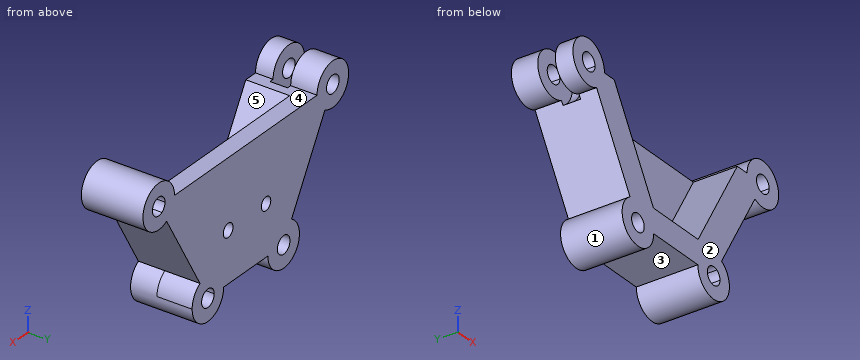
from build123d import *

# Parameters (mm, degrees)
F1_DEPTH  = 50.8
F3_DEPTH  = 76.2
F4_R      = 38.1
F1_FACE_R = 12.7
F5_DEPTH  = 12.7
F6_R      = 9.525
F6_R_2    = 9.7843029872
F7_DEPTH  = 25.401


with BuildPart() as f1:
    # F0 (on Front) → F1 (new body, symmetric)
    with BuildSketch(Plane.XZ):
        with BuildLine():
            ThreePointArc((-130.8751894546, 96.1189323328), (-190.1214960247, 111.9939323328), (-146.7501894546, 68.6226257627))
            Line((-146.7501894546, 68.6226257627), (-156.2751894546, 85.1204097048))
            ThreePointArc((-156.2751894546, 85.1204097048), (-173.6237120826, 102.4689323328), (-149.9251894546, 96.1189323328))
            Line((-149.9251894546, 96.1189323328), (-130.8751894546, 96.1189323328))
        make_face()
        with BuildLine():
            Line((-156.2751894546, 85.1204097048), (-146.7501894546, 68.6226257627))
            ThreePointArc((-146.7501894546, 68.6226257627), (-135.1288828844, 80.2439323328), (-130.8751894546, 96.1189323328))
            Line((-130.8751894546, 96.1189323328), (-149.9251894546, 96.1189323328))
            ThreePointArc((-149.9251894546, 96.1189323328), (-151.6266668265, 89.7689323328), (-156.2751894546, 85.1204097048))
        make_face()
        with BuildLine():
            Line((181.3982178505, 85.1204097048), (171.8732178505, 68.6226257627))
            ThreePointArc((171.8732178505, 68.6226257627), (203.6232178505, 68.6226257627), (219.4982178505, 96.1189323328))
            ThreePointArc((219.4982178505, 96.1189323328), (187.7482178505, 127.8689323328), (155.9982178505, 96.1189323328))
            Line((155.9982178505, 96.1189323328), (175.0482178505, 96.1189323328))
            ThreePointArc((175.0482178505, 96.1189323328), (187.7482178505, 108.8189323328), (200.4482178505, 96.1189323328))
            ThreePointArc((200.4482178505, 96.1189323328), (194.0982178505, 85.1204097048), (181.3982178505, 85.1204097048))
        make_face()
        with BuildLine():
            ThreePointArc((-79.513485802, -47.834761097), (-47.763485802, -47.834761097), (-31.888485802, -75.3310676672))
            Line((-31.888485802, -75.3310676672), (57.011514198, -75.3310676672))
            ThreePointArc((57.011514198, -75.3310676672), (72.886514198, -47.834761097), (104.636514198, -47.834761097))
            Line((104.636514198, -47.834761097), (171.8732178505, 68.6226257627))
            ThreePointArc((171.8732178505, 68.6226257627), (160.2519112804, 80.2439323328), (155.9982178505, 96.1189323328))
            Line((155.9982178505, 96.1189323328), (-130.8751894546, 96.1189323328))
            ThreePointArc((-130.8751894546, 96.1189323328), (-135.1288828844, 80.2439323328), (-146.7501894546, 68.6226257627))
            Line((-146.7501894546, 68.6226257627), (-79.513485802, -47.834761097))
        make_face()
        with BuildLine():
            Line((76.061514198, -75.3310676672), (57.011514198, -75.3310676672))
            ThreePointArc((57.011514198, -75.3310676672), (88.761514198, -107.0810676672), (120.511514198, -75.3310676672))
            ThreePointArc((120.511514198, -75.3310676672), (116.2578207681, -59.4560676672), (104.636514198, -47.834761097))
            Line((104.636514198, -47.834761097), (95.111514198, -64.3325450391))
            ThreePointArc((95.111514198, -64.3325450391), (99.760036826, -68.9810676672), (101.461514198, -75.3310676672))
            ThreePointArc((101.461514198, -75.3310676672), (88.761514198, -88.0310676672), (76.061514198, -75.3310676672))
        make_face()
        with BuildLine():
            ThreePointArc((104.636514198, -47.834761097), (72.886514198, -47.834761097), (57.011514198, -75.3310676672))
            Line((57.011514198, -75.3310676672), (76.061514198, -75.3310676672))
            ThreePointArc((76.061514198, -75.3310676672), (82.411514198, -64.3325450391), (95.111514198, -64.3325450391))
            Line((95.111514198, -64.3325450391), (104.636514198, -47.834761097))
        make_face()
        with BuildLine():
            Line((-31.888485802, -75.3310676672), (-50.938485802, -75.3310676672))
            ThreePointArc((-50.938485802, -75.3310676672), (-69.988485802, -86.3295902952), (-69.988485802, -64.3325450391))
            Line((-69.988485802, -64.3325450391), (-79.513485802, -47.834761097))
            ThreePointArc((-79.513485802, -47.834761097), (-79.513485802, -102.8273742373), (-31.888485802, -75.3310676672))
        make_face()
        with BuildLine():
            ThreePointArc((-69.988485802, -64.3325450391), (-57.288485802, -64.3325450391), (-50.938485802, -75.3310676672))
            Line((-50.938485802, -75.3310676672), (-31.888485802, -75.3310676672))
            ThreePointArc((-31.888485802, -75.3310676672), (-47.763485802, -47.834761097), (-79.513485802, -47.834761097))
            Line((-79.513485802, -47.834761097), (-69.988485802, -64.3325450391))
        make_face()
        with BuildLine():
            ThreePointArc((155.9982178505, 96.1189323328), (160.2519112804, 80.2439323328), (171.8732178505, 68.6226257627))
            Line((171.8732178505, 68.6226257627), (181.3982178505, 85.1204097048))
            ThreePointArc((181.3982178505, 85.1204097048), (176.7496952225, 89.7689323328), (175.0482178505, 96.1189323328))
            Line((175.0482178505, 96.1189323328), (155.9982178505, 96.1189323328))
        make_face()
    extrude(amount=F1_DEPTH, both=True)

    # F2 (on face) → F3 (cut)
    with BuildSketch(Plane.XZ.offset(50.8)):
        Polygon((136.4217789196, 96.1189323328), (-111.2987505236, 96.1189323328), (-32.3154252183, -40.6842000468), (57.4384536142, -40.6842000468), align=None)
    extrude(amount=-F3_DEPTH, mode=Mode.SUBTRACT)

    # F4 (on Front) + F1_face (on face) → F5 (cut, symmetric)
    with BuildSketch(Plane.XZ):
        with Locations((-162.6251894546, 96.1189323328)):
            Circle(F4_R)
    with BuildSketch(Plane(origin=(12.561514198, -50.8, 21.3503423812), x_dir=(1, 0, 0), z_dir=(0, -1, 0))):
        with BuildLine():
            Line((-123.8602647216, 74.7685899517), (-143.4367036526, 74.7685899517))
            ThreePointArc((-143.4367036526, 74.7685899517), (-202.6830102227, 90.6435899517), (-159.3117036526, 47.2722833815))
            Line((-159.3117036526, 47.2722833815), (-92.075, -69.1851034782))
            ThreePointArc((-92.075, -69.1851034782), (-92.075, -124.1777166185), (-44.45, -96.6814100483))
            Line((-44.45, -96.6814100483), (44.45, -96.6814100483))
            ThreePointArc((44.45, -96.6814100483), (92.075, -124.1777166185), (92.075, -69.1851034782))
            Line((92.075, -69.1851034782), (159.3117036526, 47.2722833815))
            ThreePointArc((159.3117036526, 47.2722833815), (202.6830102227, 90.6435899517), (143.4367036526, 74.7685899517))
            Line((143.4367036526, 74.7685899517), (123.8602647216, 74.7685899517))
            Line((123.8602647216, 74.7685899517), (44.8769394163, -62.0345424279))
            Line((44.8769394163, -62.0345424279), (-44.8769394163, -62.0345424279))
            Line((-44.8769394163, -62.0345424279), (-123.8602647216, 74.7685899517))
        make_face()
        with Locations((-76.2, -96.6814100483)):
            Circle(F1_FACE_R, mode=Mode.SUBTRACT)
        with Locations((76.2, -96.6814100483)):
            Circle(F1_FACE_R, mode=Mode.SUBTRACT)
        with Locations((-175.1867036526, 74.7685899517)):
            Circle(F1_FACE_R, mode=Mode.SUBTRACT)
        with Locations((175.1867036526, 74.7685899517)):
            Circle(F1_FACE_R, mode=Mode.SUBTRACT)
    extrude(amount=F5_DEPTH, both=True, mode=Mode.SUBTRACT)

    # F6 (on face) → F7 (cut, through all)
    with BuildSketch(Plane.XZ.offset(-25.4)):
        with Locations((-28.1673731094, -2.5842000468)):
            Circle(F6_R)
        with Locations((48.0326268906, -2.5842000468)):
            Circle(F6_R_2)
    extrude(amount=-F7_DEPTH, mode=Mode.SUBTRACT)


solid = f1.part
For this review, take the finished solid that the model builds, in its own axes (mm). Face numbers are marked on the shaded views. A direction names the side the tool comes from. Coordinates: 2 decimals unless noted, no trailing zeros. Loops run counter-clockwise (first coordinate to the right, second up) from the corner with the lowest first, then second, coordinate; pieces in that order, holes last. Notation, with made-up numbers: (21, -12.75) - (68, -12.75) arc R18 cw to (68, -8.75) - close; hole circle Ø1 at (24, 22.25). An arc over 180 degrees is marked (long way). Use a Markdown table: item, result. Add a question column.
Item 1: Insertion check: pin 1 Ø8 at (y, z) = (-12, -24.5) entering from +X; pin 2 Ø8 at (x, y) = (-145.5, -17.5) entering from -Z; pin 3 Ø25 at (x, z) = (-28.17, -2.58) entering from +Y; pin 4 Ø1 at (x, y) = (-40.5, 28.5) entering from -Z. Each pin has a flat end and moves straight along its axis. Give the tip position at first contact, or say it passes through.
Item 2: We need section D-D (z = 104.5). Give the boundary of the cut face in (x, y), and give its area (3 significant figures).
Item 3: We need section B-B (y = -29). Give the boundary of the cut face in (x, z).
Item 4: Mouldability with a two-part tool opening along X and no side actions: class the marked faces 1 and 2 as pulls with the +X half, pulls with the -X half, needs draft (parallel to the pull), parting line crosses it, or undercut.
Item 5: We need section A-A (y = -4). Give the boundary of the cut face in (x, z), and give its area (3 significant figures).
Item 6: For line 1 (X direction, y = -30, z = 86.5); line 2 (Y direction, x = 52, z = 29); line 3 (X direction, y = 29.5, z = 4.5), list the stretches that pass through material, from the lowest coordinate up.
Item 7: We need section C-C (x = 88). Give the boundary of the cut face in (y, z).
Item 8: Tool access review of the marked faces 3, 4 and 5: name each direction out of +Z, -Z, +X, -X, +Y, -Y from which nothing blocks a thin tool from reaching the whole face with its end or side.
Results list:
| question | item | result |
|---|---|---|
| 1 | pin 1 | stops at x = 120.42 |
| 1 | pin 2 | stops at z = 59.53 |
| 1 | pin 3 | stops at y = 50.8 |
| 1 | pin 4 | stops at z = -97.59 |
| 2 | outline | (-193.25, -38.1) - (-172.17, -38.1) - (-172.17, -12.7) - (-193.25, -12.7) - close; (-193.25, 12.7) - (-172.17, 12.7) - (-172.17, 50.8) - (-193.25, 50.8) - close; (-153.08, -38.1) - (-132, -38.1) - (-132, -12.7) - (-153.08, -12.7) - close; (-153.08, 12.7) - (-132, 12.7) - (-132, 50.8) - (-153.08, 50.8) - close; (157.12, -38.1) - (178.21, -38.1) - (178.21, 50.8) - (157.12, 50.8) - close; (197.29, -38.1) - (218.37, -38.1) - (218.37, 50.8) - (197.29, 50.8) - close |
| 2 | area | 6,430 mm^2 |
| 3 | outline | (-146.75, 68.62) - (-79.51, -47.83) arc R31.75 ccw (long way) to (-31.89, -75.33) - (57.01, -75.33) arc R31.75 ccw (long way) to (104.64, -47.83) - (171.87, 68.62) arc R31.75 ccw (long way) to (156, 96.12) - (136.42, 96.12) - (57.44, -40.68) - (-32.32, -40.68) - (-111.3, 96.12) - (-130.88, 96.12) arc R31.75 ccw (long way) to start; hole circle Ø25.4 at (-162.63, 96.12); hole circle Ø25.4 at (-63.64, -75.33); hole circle Ø25.4 at (88.76, -75.33); hole circle Ø25.4 at (187.75, 96.12) |
| 4 | face 1 | undercut |
| 4 | face 2 | needs draft |
| 5 | outline | (-143.58, 63.12) - (-79.51, -47.83) arc R31.75 ccw (long way) to (-31.89, -75.33) - (57.01, -75.33) arc R31.75 ccw (long way) to (104.64, -47.83) - (171.87, 68.62) arc R31.75 ccw (long way) to (156, 96.12) - (136.42, 96.12) - (57.44, -40.68) - (-32.32, -40.68) - (-111.3, 96.12) - (-124.53, 96.12) arc R38.1 cw to start; hole circle Ø25.4 at (-63.64, -75.33); hole circle Ø25.4 at (88.76, -75.33); hole circle Ø25.4 at (187.75, 96.12) |
| 5 | area | 24,600 mm^2 |
| 6 | line 1 | x = -192.88 to -170.92, -154.33 to -105.75, 130.87 to 179.46, 196.04 to 218.01 |
| 6 | line 2 | y = 25.4 to 50.8 |
| 6 | line 3 | x = -109.73 to -34.53, -21.8 to 41.28, 54.78 to 134.85 |
| 7 | outline | (-38.1, -107.07) - (50.8, -107.07) - (50.8, -88.01) - (-38.1, -88.01) - close; (-38.1, -62.65) - (50.8, -62.65) - (50.8, 96.12) - (25.4, 96.12) - (25.4, 12.25) - (-38.1, 12.25) - close |
| 8 | face 3 | -Z, +Y, -Y |
| 8 | face 4 | +Z, +Y, -Y |
| 8 | face 5 | +Z, -Y |
